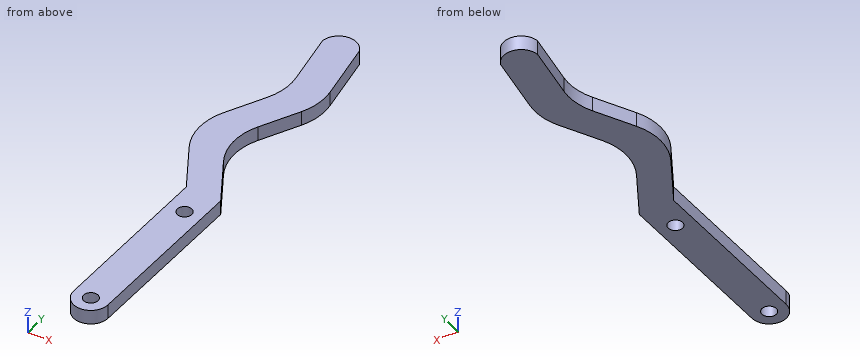
```python
from build123d import *

# Parameters (mm, degrees)
SKETCH_1_R      = 2.5
EXTRUDE_1_DEPTH = 5


with BuildPart() as part:
    # Эскиз1 → Вытянуть1 (new body)
    with BuildSketch(Plane.XY):
        with BuildLine():
            Line((-5.996779713, 0.196552972), (-5.056999721, 59.443873761))
            Line((-5.056999721, 59.443873761), (-14.520173102, 75.715501286))
            ThreePointArc((-14.520173102, 75.715501286), (-17.226120819, 85.311611147), (-14.963001631, 95.021697091))
            Line((-14.963001631, 95.021697091), (-8.160722176, 108.059141137))
            ThreePointArc((-8.160722176, 108.059141137), (-6.152874831, 114.092941719), (-6.140599008, 120.452033615))
            Line((-6.140599008, 120.452033615), (-9.157402478, 139.420199329))
            ThreePointArc((-9.157402478, 139.420199329), (-3.940932329, 144.75283841), (2.549919095, 141.076230168))
            Line((2.549919095, 141.076230168), (5.89519306, 120.042804706))
            ThreePointArc((5.89519306, 120.042804706), (5.882917236, 113.68371281), (3.875069891, 107.649912228))
            Line((3.875069891, 107.649912228), (-2.87016044, 94.721810171))
            ThreePointArc((-2.87016044, 94.721810171), (-5.133279628, 85.011724227), (-2.42733191, 75.415614366))
            Line((-2.42733191, 75.415614366), (6.976825569, 59.245462816))
            Line((6.976825569, 59.245462816), (6, 0))
            ThreePointArc((6, 0), (-0.098289675, -5.999194874), (-5.996779713, 0.196552972))
        make_face()
        Circle(SKETCH_1_R, mode=Mode.SUBTRACT)
        with Locations((0.896058218, 49.222155117)):
            Circle(SKETCH_1_R, mode=Mode.SUBTRACT)
    extrude(amount=EXTRUDE_1_DEPTH)


solid = part.part
```
The listing builds one solid part. Answer for the finished solid, in the listing's coordinates (mm). Give positions to 0.01 mm unless a question says otherwise; leave off trailing zeros. Write each loop counter-clockwise with the first axis right and the second up, starting at its lowest first coordinate (ties: lowest second). Pieces come first, ordered by that corner, then holes. Notation, with made-up numbers: (45.5, 10) -> (104.5, 10) arc R25 ccw to (104.5, 29) -> close; hole circle Ø1 at (30, 38.5). An arc over 180 degrees is marked (long way). Write item = value, one per line. Start each with the question number.
1) The part is cut by section C-C, the plane y = 126. Determine the outline of the cut face in (x, z).
2) The part is cut by section D-D, the plane y = 40. Determine the outline of the cut face in (x, z).
3) Each of these flat-tipped pins is pushed along its axis until it touches: pin 1 (1.5 mm diameter, centred on y = 50, z = 4, fed in from +X); pin 2 (3 mm diameter, centred on x = -12, z = 1, fed in from +Y). Where does it stop, or does it pass through?
4) The part is cut by section B-B, the plane z = 3.1. Determine the outline of the cut face in (x, y), and give its area (3 significant figures).
5) Straight lines are drawn through the part: line 1 along Y through (x, z) = (0, 3.2); line 2 along Y through (x, z) = (-0.5, 1.65); line 3 along X through (y, z) = (51.5, 2.25). For each, find the intervals that lie inside material, in ascending order.
6) The part is cut by section A-A, the plane x = 0. Determine the outline of the cut face in (y, z), and give its area (3 significant figures).
Solutions:
q1.outline = (-7.02, 0) -> (4.95, 0) -> (4.95, 5) -> (-7.02, 5) -> close
q2.outline = (-5.37, 0) -> (6.66, 0) -> (6.66, 5) -> (-5.37, 5) -> close
q3.pin_1 = 6.84
q3.pin_2 = 103.58
q4.outline = (-14.96, 95.02) arc R20 ccw to (-14.52, 75.72) -> (-5.06, 59.44) -> (-6, 0.2) arc R6 ccw (long way) to (6, 0) -> (6.98, 59.25) -> (-2.43, 75.42) arc R20 cw to (-2.87, 94.72) -> (3.88, 107.65) arc R20 ccw to (5.9, 120.04) -> (2.55, 141.08) arc R6.12 ccw to (-9.16, 139.42) -> (-6.14, 120.45) arc R20 cw to (-8.16, 108.06) -> close; hole circle Ø5 at (0, 0); hole circle Ø5 at (0.9, 49.22)
q4.area = 1,750 mm²
q5.line_1 = -6 to -2.5, 2.5 to 46.89, 51.56 to 71.24, 100.22 to 143.98
q5.line_2 = -5.98 to -2.45, 2.45 to 47.15, 51.3 to 72.1, 99.26 to 144.24
q5.line_3 = -5.18 to -0.13, 1.93 to 6.85
q6.outline = (-6, 0) -> (-2.5, 0) -> (-2.5, 5) -> (-6, 5) -> close; (2.5, 0) -> (46.89, 0) -> (46.89, 5) -> (2.5, 5) -> close; (51.56, 0) -> (71.24, 0) -> (71.24, 5) -> (51.56, 5) -> close; (100.22, 0) -> (143.98, 0) -> (143.98, 5) -> (100.22, 5) -> close
q6.area = 557 mm²
